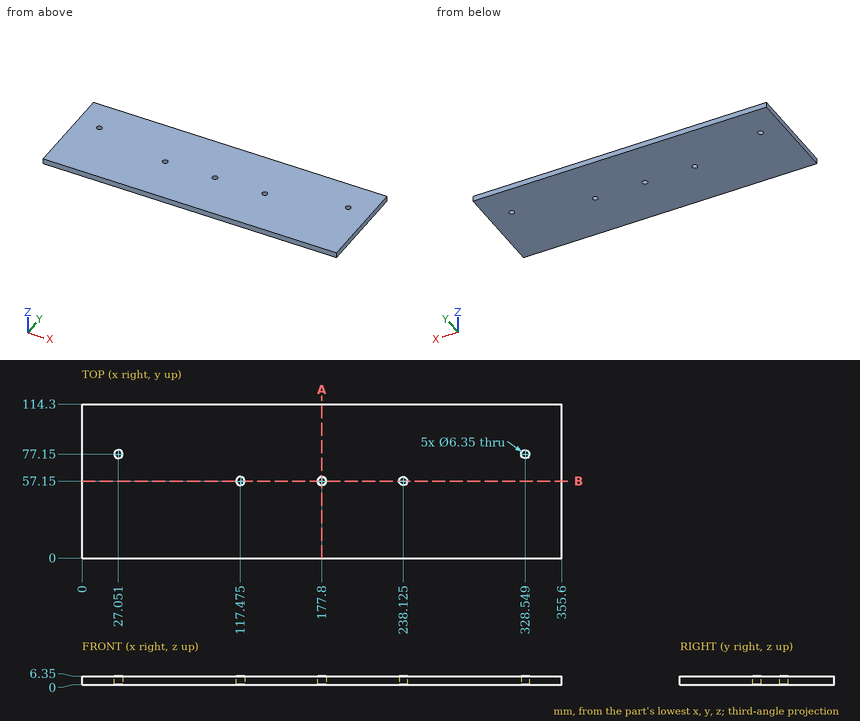
For this review, use the dimensioned drawing (mm, ordinates from the lowest corner) and the shaded views. Give positions to 0.01 mm unless a question says otherwise; leave off trailing zeros. Order: outer loops, then holes, each group sorted by start corner. A loop starts at its lowest first (then second) coordinate and runs counter-clockwise, first axis right, second up.
1. For pin 1 Ø10 at (x, y) = (27.051, 77.15) entering from -Z, flat-tipped, find the tip position at first contact; note if it passes through.
Solution:
pin 1: stops at z = 0
2. To check wall thickness, follow L1, parallel to X at y = 77.15, z = 3.5; L2, parallel to Y at x = 177.8, z = 3.5 (3 decimals); L3, parallel to Y at x = 175, z = 2.5. State the ranges of each line that lie inside material, in increasing order.
Solution:
L1: x = 0 to 23.88, 30.23 to 325.37, 331.72 to 355.6
L2: y = 0 to 53.975, 60.325 to 114.3
L3: y = 0 to 55.65, 58.65 to 114.3
3. Add section B-B, the plane y = 57.15. State the section outline as (x, z) points (3 decimals), then the cut area to 3 significant figures.
Solution:
outline: (0, 0) - (114.3, 0) - (114.3, 6.35) - (0, 6.35) - close; (120.65, 0) - (174.625, 0) - (174.625, 6.35) - (120.65, 6.35) - close; (180.975, 0) - (234.95, 0) - (234.95, 6.35) - (180.975, 6.35) - close; (241.3, 0) - (355.6, 0) - (355.6, 6.35) - (241.3, 6.35) - close
area: 2,140 mm2
4. Add section A-A, the plane x = 177.8. State the section outline as (y, z) points (3 decimals).
Solution:
outline: (0, 0) - (53.975, 0) - (53.975, 6.35) - (0, 6.35) - close; (60.325, 0) - (114.3, 0) - (114.3, 6.35) - (60.325, 6.35) - close
